```python
from build123d import *

# Parameters (mm, degrees)
CROQUIS1_W              = 50.8
CROQUIS1_H              = 76.2
SALIENTE_EXTRUIR1_DEPTH = 18
CROQUIS2_W              = 50.8
CROQUIS2_H              = 76.2
CROQUIS2_W_2            = 46.12
CROQUIS2_H_2            = 71.52
CROQUIS2_W_3            = 38.8
CROQUIS2_H_3            = 64.2
CORTAR_EXTRUIR1_DEPTH   = 15
CORTAR_EXTRUIR8_DEPTH   = 15
SALIENTE_EXTRUIR3_DEPTH = 41.5
CORTAR_EXTRUIR9_DEPTH   = 51.5
CORTAR_EXTRUIR10_DEPTH  = 51.5
SALIENTE_EXTRUIR4_DEPTH = 16
CORTAR_EXTRUIR11_DEPTH  = 16.5
REDONDEO3_R             = 2
REDONDEO4_R             = 1
CROQUIS15_W             = 48.12
CROQUIS15_H             = 10
CORTAR_EXTRUIR12_DEPTH  = 15
CROQUIS16_W             = 8
CROQUIS16_H             = 1.5
CORTAR_EXTRUIR13_DEPTH  = 2


with BuildPart() as part:
    # Croquis1 → Saliente-Extruir1 (new body)
    with BuildSketch(Plane.XY):
        Rectangle(CROQUIS1_W, CROQUIS1_H)
    extrude(amount=SALIENTE_EXTRUIR1_DEPTH)

    # Croquis2 → Cortar-Extruir1 (cut)
    # profile 1 of 2: a face of its own
    with BuildSketch(Plane.XY.offset(18)):
        Rectangle(CROQUIS2_W, CROQUIS2_H)
        Rectangle(CROQUIS2_W_2, CROQUIS2_H_2, mode=Mode.SUBTRACT)
    # profile 2 of 2: a face of its own
    with BuildSketch(Plane.XY.offset(18)):
        Rectangle(CROQUIS2_W_3, CROQUIS2_H_3)
    extrude(amount=-CORTAR_EXTRUIR1_DEPTH, mode=Mode.SUBTRACT)

    # Croquis6 → Cortar-Extruir8 (cut)
    with BuildSketch(Plane.XY.offset(18)):
        Polygon((-23.06, 35.76), (-8.06, 35.76), (-8.06, 32.1), (-19.4, 32.1), (-19.4, 20.76), (-23.06, 20.76), align=None)
        Polygon((23.06, 35.76), (8.06, 35.76), (8.06, 32.1), (19.4, 32.1), (19.4, 20.76), (23.06, 20.76), align=None)
        Polygon((-23.06, -35.76), (-23.06, -20.76), (-19.4, -20.76), (-19.4, -32.1), (-8.06, -32.1), (-8.06, -35.76), align=None)
        Polygon((23.06, -35.76), (8.06, -35.76), (8.06, -32.1), (19.4, -32.1), (19.4, -20.76), (23.06, -20.76), align=None)
    extrude(amount=-CORTAR_EXTRUIR8_DEPTH, mode=Mode.SUBTRACT)

    # Croquis10 → Saliente-Extruir3 (add)
    with BuildSketch(Plane(origin=(0, -20.76, 0), x_dir=(-1, 0, 0), z_dir=(0, -1, 0))):
        Polygon((23.06, -18), (24.06, -18), (23.06, -3), align=None)
        Polygon((-23.06, -18), (-24.06, -18), (-23.06, -3), align=None)
    extrude(amount=-SALIENTE_EXTRUIR3_DEPTH)

    # Croquis11 → Cortar-Extruir9 (cut)
    with BuildSketch(Plane.XZ.offset(20.76)):
        Polygon((-19.4, 18), (-21.56, 18), (-20.56, 3), (-19.4, 3), align=None)
    extrude(amount=-CORTAR_EXTRUIR9_DEPTH, mode=Mode.SUBTRACT)

    # Croquis12 → Cortar-Extruir10 (cut)
    with BuildSketch(Plane.XZ.offset(20.76)):
        Polygon((19.4, 18), (19.4, 3), (20.56, 3), (21.56, 18), align=None)
    extrude(amount=-CORTAR_EXTRUIR10_DEPTH, mode=Mode.SUBTRACT)

    # Croquis13 → Saliente-Extruir4 (add)
    with BuildSketch(Plane(origin=(8.06, 0, 0), x_dir=(0, 0, -1), z_dir=(1, 0, 0))):
        Polygon((-18, -35.76), (-18, -37.76), (-3, -35.76), align=None)
        Polygon((-18, 35.76), (-18, 37.76), (-3, 35.76), align=None)
    extrude(amount=-SALIENTE_EXTRUIR4_DEPTH)

    # Croquis14 → Cortar-Extruir11 (cut)
    with BuildSketch(Plane(origin=(8.06, 0, 0), x_dir=(0, 0, -1), z_dir=(1, 0, 0))):
        Polygon((-3, -32.1), (-18, -32.1), (-18, -35.26), (-3, -33.26), align=None)
        Polygon((-18, 32.1), (-18, 35.26), (-3, 33.26), (-3, 32.1), align=None)
    extrude(amount=-CORTAR_EXTRUIR11_DEPTH, mode=Mode.SUBTRACT)

    # Redondeo3
    redondeo3_edges = [part.edges().sort_by_distance(p)[0] for p in [
        (-25.4, 38.1, 1.5),
        (25.4, 38.1, 1.5),
        (25.4, -38.1, 1.5),
        (-25.4, -38.1, 1.5),
    ]]
    fillet(redondeo3_edges, radius=REDONDEO3_R)

    # Redondeo4
    redondeo4_edges = [part.edges().sort_by_distance(p)[0] for p in [
        (0, 38.1, 0),
        (-25.4, 0, 0),
        (25.4, 0, 0),
        (0, -38.1, 0),
        (24.814213562, -37.514213562, 0),
        (-24.814213562, -37.514213562, 0),
        (-24.814213562, 37.514213562, 0),
        (24.814213562, 37.514213562, 0),
    ]]
    fillet(redondeo4_edges, radius=REDONDEO4_R)

    # Croquis15 → Cortar-Extruir12 (cut)
    with BuildSketch(Plane.XY.offset(18)):
        with Locations((0, -0.01)):
            Rectangle(CROQUIS15_W, CROQUIS15_H)
    extrude(amount=-CORTAR_EXTRUIR12_DEPTH, mode=Mode.SUBTRACT)

    # Croquis16 → Cortar-Extruir13 (cut)
    with BuildSketch(Plane.XZ.offset(38.1)):
        with Locations((0, 2.25)):
            Rectangle(CROQUIS16_W, CROQUIS16_H)
    extrude(amount=-CORTAR_EXTRUIR13_DEPTH, mode=Mode.SUBTRACT)


solid = part.part
```
The listing builds one solid part. Answer for the finished solid, in the listing's coordinates (mm). A direction names the side the tool comes from. Give positions to 0.01 mm unless a question says otherwise; leave off trailing zeros. Loops run counter-clockwise (first coordinate to the right, second up) from the corner with the lowest first, then second, coordinate; pieces in that order, holes last. Notation, with made-up numbers: M 10,5.25 L 42,5.25 A16 ccw 42,27.25 Z; hole C 19.5,-31 d5. An arc over 180 degrees is marked long. One line per item, written item: value.
1. Section A-A on z = 12.75 is taken. State how many separate pieces and enclosed holes the cut face has, plus the area to 3 significant figures.
Found:
separate pieces: 6
enclosed holes: 0
area: 238 mm^2
2. For faces 5 (the face through (-7.94, -36.5, 12.3)), 6 (the face through (-4, -37, 2)), 7 (the face through (-23.567, -12.995, 10.605)), 8 (the face through (0.172, 36.774, 10.605)), determine the directions among +Z, -Z, +X, -X, +Y, -Y from which every point of the face is accessible in a straight line to the end or side of a thin tool.
Found:
face 5: +Z, -X, -Y
face 6: -Y
face 7: -X, +Y, -Y
face 8: +X, -X, +Y
3. Section B-B on x = 6.5 is taken. Determine the outline of the cut face in (y, z), plus the area to 3 significant figures.
Found:
outline: M -38.1,1 A1 ccw -37.1,0 L 37.1,0 A1 ccw 38.1,1 L 38.1,3 L 35.76,3 L 37.76,18 L 35.26,18 L 33.26,3 L -33.26,3 L -35.26,18 L -37.76,18 L -35.76,3 L -38.1,3 Z
area: 303 mm^2
4. Each of these flat-tipped pins is pushed along its axis until it touches: P1, Ø4, axis at y = -18, z = 7, coming from the +X side; P2, Ø0.8, axis at x = -22.5, z = 14, coming from the +Y side; P3, Ø0.6, axis at y = 36.5, z = 8.5, coming from the -X side; P4, Ø6, axis at y = -1, z = 9.5, coming from the +X side. Where does it stop, or does it pass through?
Found:
P1: x = 23.46
P2: y = 20.76
P3: x = -7.94
P4: through
5. Find the intervals of material crossed by probe 1 along Y at (x, z) = (-22, 13); probe 2 along Z at (x, y) = (17, 28); probe 3 along Y at (x, z) = (2, 2), in increasing order.
Found:
probe 1: -20.76 to -5.01, 4.99 to 20.76
probe 2: 0 to 3
probe 3: -36.1 to 38.1
6. Section C-C on y = 30 is taken. Determine the outline of the cut face in (x, z).
Found:
outline: M -25.4,1 A1 ccw -24.4,0 L 24.4,0 A1 ccw 25.4,1 L 25.4,3 L -25.4,3 Z
7. For a pull along X with two mould halves and no side action, classify faces 1 (the face through (21.053, -12.995, 10.395)), 2 (the face through (21.053, 12.765, 10.395)), 3 (the face through (24.8, 37.53, 2.01)), 4 (the face through (-0.3, -38.1, 1.3)) as pulls with the +X half, pulls with the -X half, needs draft (parallel to the pull), parting line crosses it, or undercut.
Found:
face 1: undercut
face 2: undercut
face 3: pulls with the +X half
face 4: needs draft
